```python
from build123d import *

# Parameters (mm, degrees)
BOSS_EXTRUDE1_DEPTH = 10
SKETCH1_4_W         = 16.4
SKETCH1_4_H         = 37.6
BOSS_EXTRUDE2_DEPTH = 4
SKETCH3_W           = 18
SKETCH3_H           = 5
CUT_EXTRUDE2_DEPTH  = 41.099875312
FILLET1_R           = 2
FILLET2_R           = 1


with BuildPart() as part:
    # Sketch1 → Boss-Extrude1 (new body)
    with BuildSketch(Plane(origin=(0, 0, 0), x_dir=(1, 0, 0), z_dir=(0, 1, 0))):
        with BuildLine():
            Line((-9, -21.5), (9, -21.5))
            ThreePointArc((9, -21.5), (10.414213562, -20.914213562), (11, -19.5))
            Line((11, -19.5), (11, 19.5))
            ThreePointArc((11, 19.5), (10.414213562, 20.914213562), (9, 21.5))
            Line((9, 21.5), (-9, 21.5))
            ThreePointArc((-9, 21.5), (-10.414213562, 20.914213562), (-11, 19.5))
            Line((-11, 19.5), (-11, -19.5))
            ThreePointArc((-11, -19.5), (-10.414213562, -20.914213562), (-9, -21.5))
        make_face()
    extrude(amount=BOSS_EXTRUDE1_DEPTH)

    # Sketch1<4> → Boss-Extrude2 (add)
    with BuildSketch(Plane(origin=(0, 0, 0), x_dir=(1, 0, 0), z_dir=(0, 1, 0))):
        Rectangle(SKETCH1_4_W, SKETCH1_4_H)
    extrude(amount=-BOSS_EXTRUDE2_DEPTH)

    # Sketch3 → Cut-Extrude2 (cut, through all)
    with BuildSketch(Plane(origin=(-11, 0, 10.5), x_dir=(0, 0, -1), z_dir=(1, 0, 0))):
        with Locations((10.5, 5)):
            Rectangle(SKETCH3_W, SKETCH3_H)
    extrude(amount=CUT_EXTRUDE2_DEPTH, mode=Mode.SUBTRACT)

    # Fillet1
    fillet1_edges = [part.edges().sort_by_distance(p)[0] for p in [
        (-11, 2.5, 0),
        (11, 2.5, 0),
    ]]
    fillet(fillet1_edges, radius=FILLET1_R)

    # Fillet2
    fillet2_edges = [part.edges().sort_by_distance(p)[0] for p in [
        (10.414213562, 10, -20.914213562),
        (11, 10, 0),
        (10.414213562, 10, 20.914213562),
        (0, 10, 21.5),
        (-10.414213562, 10, 20.914213562),
        (-11, 10, 0),
        (-10.414213562, 10, -20.914213562),
        (0, 10, -21.5),
    ]]
    fillet(fillet2_edges, radius=FILLET2_R)


solid = part.part
```
Can you work these out from the model? Positions are in its coordinate system, mm. A direction names the side the tool comes from. Give positions to 0.01 mm unless a question says otherwise; leave off trailing zeros. Loops run counter-clockwise (first coordinate to the right, second up) from the corner with the lowest first, then second, coordinate; pieces in that order, holes last. Notation, with made-up numbers: M 78.5,0 L 123.5,0 A20 cw 123.5,8 Z; hole C 13.25,-10.5 d6. An arc over 180 degrees is marked long. Answer in a Markdown table with one row per item.
1. Suppose I cut it at C-C on x = -5.25. Write out the boundary of the cut face in (y, z).
Taken from the geometry:
| item | result |
|---|---|
| outline | M -4,-18.8 L 0,-18.8 L 0,-21.5 L 9,-21.5 A1 ccw 10,-20.5 L 10,20.5 A1 ccw 9,21.5 L 0,21.5 L 0,18.8 L -4,18.8 Z; hole M 2.5,-9 L 7.5,-9 L 7.5,9 L 2.5,9 Z |
2. Thinking about a two-plate mould opening in Y: for faces 6 (the cylindrical face through (-0.126, 9.699, -21.215)), 7 (the flat face through (0, 7.5, 0)), 8 (the flat face through (11, 8, 0)), which applies, released by +Y, released by -Y, zero draft, split by the parting line, or undercut?
Taken from the geometry:
| item | result |
|---|---|
| face 6 | released by +Y |
| face 7 | undercut |
| face 8 | zero draft |
3. If I drill on line 1 along Z through (x, y) = (2.75, 3.25); line 2 along Y through (x, z) = (-6, 2); line 3 along Y through (x, z) = (-8.5, 1), over which ranges is the centre line in solid material (lowest first)?
Taken from the geometry:
| item | result |
|---|---|
| line 1 | z = -21.5 to -9, 9 to 21.5 |
| line 2 | y = -4 to 2.5, 7.5 to 10 |
| line 3 | y = 0 to 2.5, 7.5 to 10 |
4. Suppose I cut it at A-A on y = 4.5. Write out the boundary of the cut face in (x, z), plus the area to 3 significant figures.
Taken from the geometry:
| item | result |
|---|---|
| outline | M -11,-19.5 A2 ccw -9,-21.5 L 9,-21.5 A2 ccw 11,-19.5 L 11,-9 L -11,-9 Z; M -11,9 L 11,9 L 11,19.5 A2 ccw 9,21.5 L -9,21.5 A2 ccw -11,19.5 Z |
| area | 547 mm² |
5. Which directions (+Z, -Z, +X, -X, +Y, -Y) give clear straight access to the entire face, cutting with the end or side of a thin tool? Please do faces 1 (the cylindrical face through (10.43, 1.9, -0.13)), 2 (the flat face through (-8.2, -2, 0)), 3 (the cylindrical face through (-10.43, 1.9, -0.13)), 4 (the flat face through (0, -2, 18.8)), 5 (the flat face through (8.2, -2, 0)).
Taken from the geometry:
| item | result |
|---|---|
| face 1 | +X |
| face 2 | +Z, -Z, -X, -Y |
| face 3 | -X |
| face 4 | +Z, +X, -X, -Y |
| face 5 | +Z, -Z, +X, -Y |
6. Suppose I cut it at B-B on z = 6.5. Write out the boundary of the cut face in (x, y).
Taken from the geometry:
| item | result |
|---|---|
| outline | M -11,0 L -8.2,0 L -8.2,-4 L 8.2,-4 L 8.2,0 L 11,0 L 11,0.5 A2 ccw 9,2.5 L -9,2.5 A2 ccw -11,0.5 Z; M -11,7.5 L 11,7.5 L 11,9 A1 ccw 10,10 L -10,10 A1 ccw -11,9 Z |
7. For pin 1 Ø3 at (y, z) = (-3, -4.5) entering from +X; pin 2 Ø3 at (x, y) = (-4, -3) entering from +Z; pin 3 Ø3 at (y, z) = (-2, 6.5) entering from -X, each with a flat end and sliding along its axis, tell me the tip position at first contact or that it passes through.
Taken from the geometry:
| item | result |
|---|---|
| pin 1 | stops at x = 8.2 |
| pin 2 | stops at z = 18.8 |
| pin 3 | stops at x = -8.2 |
8. Suppose I cut it at D-D on z = -18. Write out the boundary of the cut face in (x, y), plus the area to 3 significant figures.
Taken from the geometry:
| item | result |
|---|---|
| outline | M -11,0 L -8.2,0 L -8.2,-4 L 8.2,-4 L 8.2,0 L 11,0 L 11,9 A1 ccw 10,10 L -10,10 A1 ccw -11,9 Z |
| area | 285 mm² |
